The listing builds one solid part. Answer for the finished solid, in the listing's coordinates (mm). Give positions to 0.01 mm unless a question says otherwise; leave off trailing zeros. Write each loop counter-clockwise with the first axis right and the second up, starting at its lowest first coordinate (ties: lowest second). Pieces come first, ordered by that corner, then holes. Notation, with made-up numbers: M 23,60 L 38,60 A26 ccw 38,80 Z; hole C -1.5,-27 d6. An arc over 180 degrees is marked long. Return JSON: item names as keys, results as strings.
from build123d import *

# Parameters (mm, degrees)
SKETCH1_R           = 3.82
BOSS_EXTRUDE1_DEPTH = 0.43
FILLET1_R           = 2


with BuildPart() as part:
    # Sketch1 → Boss-Extrude1 (new body)
    with BuildSketch(Plane.XY):
        Circle(SKETCH1_R)
        with BuildLine():
            Line((-3.2, -2.086240638), (-3.2, -6.586240638))
            Line((-3.2, -6.586240638), (3.2, -6.586240638))
            Line((3.2, -6.586240638), (3.2, -2.086240638))
            ThreePointArc((3.2, -2.086240638), (0, -3.82), (-3.2, -2.086240638))
        make_face()
    extrude(amount=BOSS_EXTRUDE1_DEPTH)

    # Fillet1
    fillet1_edges = [part.edges().sort_by_distance(p)[0] for p in [
        (3.2, -2.086240638, 0.215),
        (-3.2, -2.086240638, 0.215),
    ]]
    fillet(fillet1_edges, radius=FILLET1_R)


solid = part.part
Item 1: A cutting plane is placed at B-B, the plane y = -3.75. Write down the section's boundary in (x, z).
Geometry results:
{"outline": "M -3.2,0 L 3.2,0 L 3.2,0.43 L -3.2,0.43 Z"}
Item 2: A cutting plane is placed at A-A, the plane z = 0.3. Write down the section's boundary in (x, y), plus the area to 3 significant figures.
Geometry results:
{"outline": "M -3.41,-1.72 A2 cw -3.2,-2.61 L -3.2,-6.59 L 3.2,-6.59 L 3.2,-2.61 A2 cw 3.41,-1.72 A3.82 ccw long Z", "area": "66.9 mm2"}
Item 3: Find the intervals of material crossed by line 1 (X direction, y = -4, z = 0.1); line 2 (Y direction, x = -0.5, z = 0.25); line 3 (X direction, y = 0.5, z = 0.2), in increasing order.
Geometry results:
{"line 1": "x = -3.2 to 3.2", "line 2": "y = -6.59 to 3.79", "line 3": "x = -3.79 to 3.79"}
Item 4: A cutting plane is placed at C-C, the plane x = 1.5. Write down the section's boundary in (y, z), plus the area to 3 significant figures.
Geometry results:
{"outline": "M -6.59,0 L 3.51,0 L 3.51,0.43 L -6.59,0.43 Z", "area": "4.34 mm2"}
